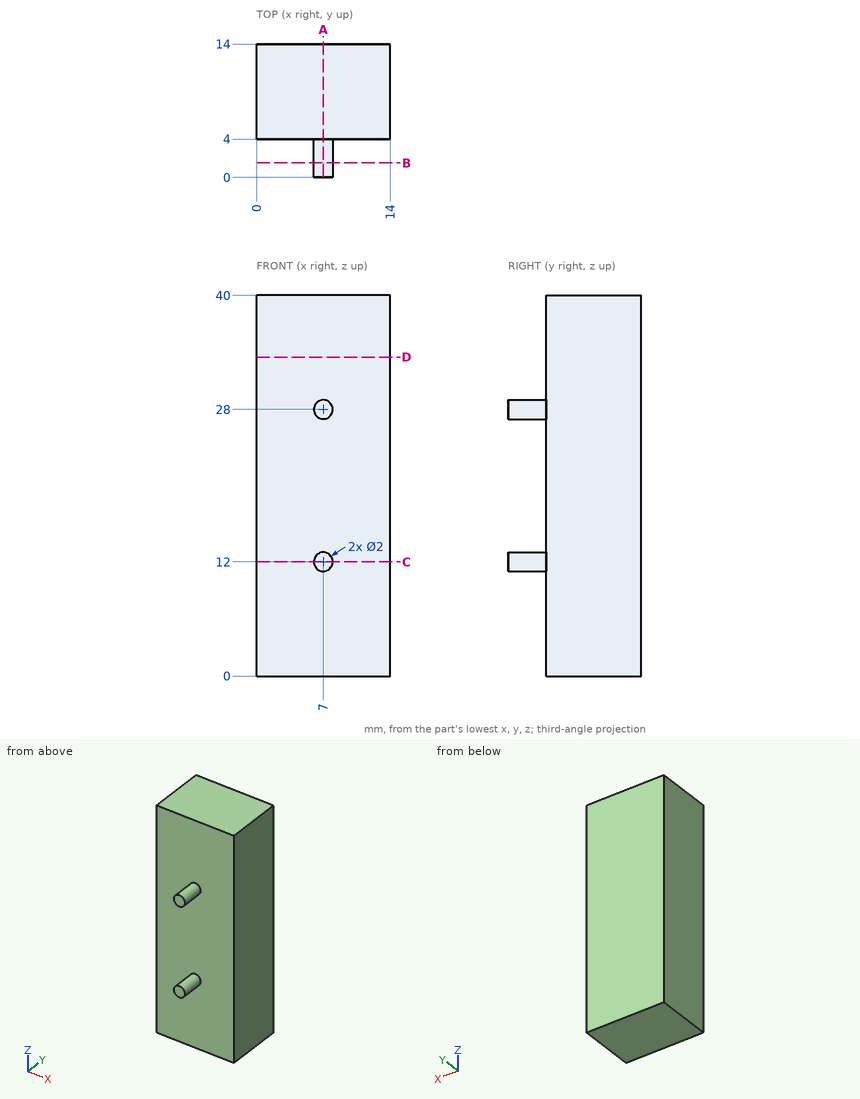
Study the drawing (mm; zero at the part's minimum x, y, z) and answer. Coordinates: 2 decimals unless noted, no trailing zeros. Write each loop counter-clockwise with the first axis right and the second up, starting at its lowest first coordinate (ties: lowest second). Pieces come first, ordered by that corner, then holes. Notation, with made-up numbers: (48, 54) -> (75, 54) arc R33 ccw to (75, 91) -> close; hole circle Ø3 at (18, -39.75). An arc over 180 degrees is marked (long way). Write each question's results on one line, items separated by ' | '. Start each with the question number.
1) A cutting plane is placed at A-A (x = 7). Determine the outline of the cut face in (y, z), then the cut area to 3 significant figures.
2) A cutting plane is placed at C-C (z = 12). Determine the outline of the cut face in (x, y), then the cut area to 3 significant figures.
3) A cutting plane is placed at D-D (z = 33.5). Determine the outline of the cut face in (x, y), then the cut area to 3 significant figures.
4) A cutting plane is placed at B-B (y = 1.5). Determine the outline of the cut face in (x, z), then the cut area to 3 significant figures.
5) Flat-ended cylindrical pins translate along their axes: pin 1 Ø1.5 at (x, z) = (4.5, 19) entering from -Y; pin 2 Ø2 at (x, y) = (7, 8) entering from -Z; pin 3 Ø1 at (x, y) = (11, 2.5) entering from -Z. Find the tip coordinate at first contact, or state that the pin passes through.
6) A straight line is drawn through the part: probe 1 along Y at (x, z) = (3.25, 14). Find the intervals that lie inside material, in ascending order.
Values follow:
1) outline: (0, 11) -> (4, 11) -> (4, 0) -> (14, 0) -> (14, 40) -> (4, 40) -> (4, 29) -> (0, 29) -> (0, 27) -> (4, 27) -> (4, 13) -> (0, 13) -> close | area: 416 mm²
2) outline: (0, 4) -> (6, 4) -> (6, 0) -> (8, 0) -> (8, 4) -> (14, 4) -> (14, 14) -> (0, 14) -> close | area: 148 mm²
3) outline: (0, 4) -> (14, 4) -> (14, 14) -> (0, 14) -> close | area: 140 mm²
4) outline: circle Ø2 at (7, 12); circle Ø2 at (7, 28) | area: 6.28 mm²
5) pin 1: y = 4 | pin 2: z = 0 | pin 3: through
6) probe 1: 4 to 14
